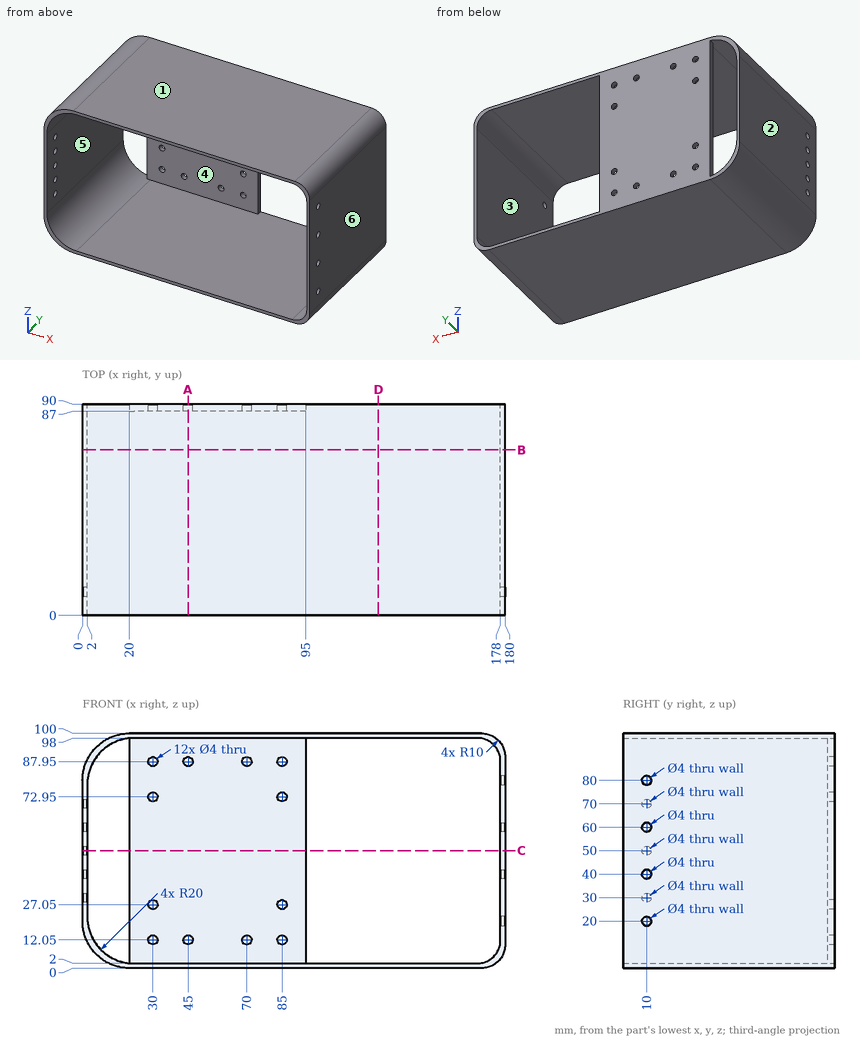
The figure shows three views and two pictorial views of one solid part (mm, origin at its lowest corner). Answer the questions. A direction names the side the tool comes from. Coordinates: 2 decimals unless noted, no trailing zeros. Loops run counter-clockwise (first coordinate to the right, second up) from the corner with the lowest first, then second, coordinate; pieces in that order, holes last.
1) Find the intervals of material crossed by L1, parallel to X at y = 83, z = 33; L2, parallel to Y at x = 1.4, z = 50; L3, parallel to Z at x = 70, y = 87.9, in increasing order.
2) Find section B-B on y = 70.5. Write down the section's boundary in (x, z), then the cut area to 3 significant figures.
3) Find section C-C on z = 50. Write down the section's boundary in (x, y), then the cut area to 3 significant figures.
4) Flat-ended cylindrical pins translate along their axes: pin 1 Ø3 at (y, z) = (10, 60) entering from +X; pin 2 Ø6.5 at (x, z) = (70, 12.05) entering from -Y; pin 3 Ø3 at (y, z) = (10, 20) entering from +X. Find the tip coordinate at first contact, or state that the pin passes through.
5) Determine the mould class of the marked faces 1, 2 and 3 for opening direction Z: pulls with the +Z half, pulls with the -Z half, needs draft (parallel to the pull), parting line crosses it, or undercut.
6) Find section A-A on x = 45. Write down the section's boundary in (y, z), then the cut area to 3 significant figures.
7) A tool of negligible diameter and unlimited length cuts with its end or side. For the marked faces 4, 5 and 6, from which of +Z, -Z, +X, -X, +Y, -Y can it reach the whole face along a straight path? Write none if from no direction.
8) Find section D-D on x = 126. Write down the section's boundary in (y, z), then the cut area to 3 significant figures.
Values:
1. L1: x = 0 to 2, 178 to 180
1. L2: y = 0 to 8, 12 to 90
1. L3: z = 0 to 10.05, 14.05 to 85.95, 89.95 to 100
2. outline: (0, 20) arc R20 ccw to (20, 0) - (170, 0) arc R10 ccw to (180, 10) - (180, 90) arc R10 ccw to (170, 100) - (20, 100) arc R20 ccw to (0, 80) - close; hole (2, 22) arc R20 ccw to (22, 2) - (168, 2) arc R10 ccw to (178, 12) - (178, 88) arc R10 ccw to (168, 98) - (22, 98) arc R20 ccw to (2, 78) - close
2. area: 1,100 mm2
3. outline: (0, 0) - (2, 0) - (2, 8) - (0, 8) - close; (0, 12) - (2, 12) - (2, 90) - (0, 90) - close; (20, 87) - (95, 87) - (95, 90) - (20, 90) - close; (178, 0) - (180, 0) - (180, 90) - (178, 90) - close
3. area: 577 mm2
4. pin 1: passes through
4. pin 2: stops at y = 87
4. pin 3: stops at x = 2.31
5. face 1: pulls with the +Z half
5. face 2: needs draft
5. face 3: undercut
6. outline: (0, 0) - (90, 0) - (90, 10.05) - (87, 10.05) - (87, 2) - (0, 2) - close; (0, 98) - (87, 98) - (87, 89.95) - (90, 89.95) - (90, 100) - (0, 100) - close; (87, 14.05) - (90, 14.05) - (90, 85.95) - (87, 85.95) - close
6. area: 624 mm2
7. face 4: -Y
7. face 5: +Y, -Y
7. face 6: +Z, -Z, +X, +Y, -Y
8. outline: (0, 0) - (90, 0) - (90, 2) - (0, 2) - close; (0, 98) - (90, 98) - (90, 100) - (0, 100) - close
8. area: 360 mm2
